Verification items for the finished model (mm, model axes). Face numbers are marked on the shaded views. A direction names the side the tool comes from. Round coordinates to 2 decimals unless told otherwise and drop trailing zeros. Order: outer loops, then holes, each group sorted by start corner. A loop starts at its lowest first (then second) coordinate and runs counter-clockwise, first axis right, second up. Notation, with made-up numbers: (36.5, 49) -> (66.5, 49) arc R20 ccw to (66.5, 75) -> close; hole circle Ø7 at (59, 46.5). An arc over 180 degrees is marked (long way). Put each result on its own line as item: value.
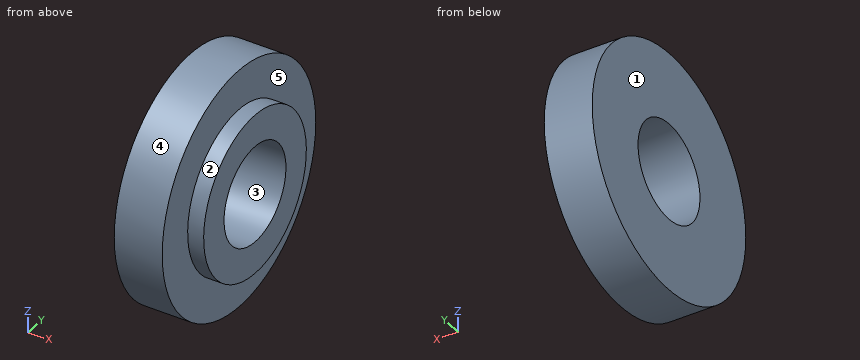
Autodesk Inventor part; units mm, degrees
ref_plane "YZ Plane" through (0, 0, 0) normal (1, 0, 0) x (0, 1, 0)
ref_plane "XZ Plane" through (0, 0, 0) normal (0, 1, 0) x (-1, 0, 0)
ref_plane "XY Plane" through (0, 0, 0) normal (0, 0, 1) x (1, 0, 0)
sketch "Sketch1" plane through (0, 0, 0) normal (1, 0, 0) x (0, 1, 0)
  circle A0 centre (0, 0) radius 3.7375
  dimension "d0" = 7.475
extrude "Extrusion1" add sketch "Sketch1" along normal blind 1.5
sketch "Sketch2" plane through (1.5, 0, 0) normal (1, 0, 0) x (0, 0, -1)
  circle A0 centre (0, 0) radius 2.5
  dimension "d4" = 5
extrude "Extrusion2" add sketch "Sketch2" along normal blind 0.5
sketch "Sketch3" plane through (2, 0, 0) normal (1, 0, 0) x (0, 0, -1)
  circle A0 centre (0, 0) radius 2.5
hole "Hole1" at (2, 0, 0) direction (-1, 0, 0) diameter 3.015 end through all
properties part number "roller"
Item 1: Section check D-D on y = 2. Record the boundary of the cut face in (x, z).
Check sheet entries:
outline: (0, -3.16) -> (1.5, -3.16) -> (1.5, -1.5) -> (2, -1.5) -> (2, 1.5) -> (1.5, 1.5) -> (1.5, 3.16) -> (0, 3.16) -> close
Item 2: Release check for a two-part mould opening along Y. For the marked faces 1, 2 and 3 record: +Y half, -Y half, draft (parallel to the pull), parting line (faces both ways), or undercut.
Check sheet entries:
face 1: draft
face 2: parting line
face 3: undercut
Item 3: Tool access check on the marked faces 4 and 5. Record the directions out of +Z, -Z, +X, -X, +Y, -Y that give a thin tool (end or side, any length) a straight path to the whole face; none if there is none.
Check sheet entries:
face 4: +X, -X
face 5: +X
Item 4: Section check A-A on y = 0. Record the boundary of the cut face in (x, z), then the cut area to 3 significant figures.
Check sheet entries:
outline: (0, -3.74) -> (1.5, -3.74) -> (1.5, -2.5) -> (2, -2.5) -> (2, -1.51) -> (0, -1.51) -> close; (0, 1.51) -> (2, 1.51) -> (2, 2.5) -> (1.5, 2.5) -> (1.5, 3.74) -> (0, 3.74) -> close
area: 7.68 mm^2
Item 5: Material ranges on L1, parallel to Z at x = 1.45, y = 0; L2, parallel to X at y = 1.5, z = 2.5; L3, parallel to Z at x = 0.2, y = -1, recorded low to high. Write a range as [from, to].
Check sheet entries:
L1: z = [-3.74, -1.51], [1.51, 3.74]
L2: x = [0, 1.5]
L3: z = [-3.6, -1.13], [1.13, 3.6]
Item 6: Section check C-C on x = 1.75. Record the boundary of the cut face in (y, z) (1 decimal), then the cut area to 3 significant figures.
Check sheet entries:
outline: circle Ø5 at (0, 0); hole circle Ø3 at (0, 0)
area: 12.5 mm^2
